from build123d import *

# Parameters (mm, degrees)
F2_SIZE  = 1.5
F3_W     = 30
F3_H     = 3
F4_DEPTH = 3.001


with BuildPart() as f1:
    # F0 (on Front) → F1 (revolve)
    with BuildSketch(Plane.XZ):
        Polygon((0, 10), (0, 15), (-3, 15), (-3, 0), (45, 0), (45, 10), (41.5, 10), (41.5, 7.5), (39.95, 7.5), (39.95, 10), align=None)
    revolve(axis=Axis((21, 0, 0), (1, 0, 0)))

    # F2
    f2_edges = [f1.edges().sort_by_distance(p)[0] for p in [
        (45, 0, -10),
        (-3, 0, -15),
    ]]
    chamfer(f2_edges, length=F2_SIZE)

    # F3 (on Right) → F4 (cut, through all)
    with BuildSketch(Plane.YZ):
        with Locations((0, 13.5)):
            Rectangle(F3_W, F3_H)
    extrude(amount=-F4_DEPTH, mode=Mode.SUBTRACT)


solid = f1.part
Input: part model. Units: mm. Frame: model coordinates. A direction names the side the tool comes from. Give positions to 0.01 mm unless a question says otherwise; leave off trailing zeros. Order: outer loops, then holes, each group sorted by start corner. A loop starts at its lowest first (then second) coordinate and runs counter-clockwise, first axis right, second up. Notation, with made-up numbers: (-31, 42.25) - (-6, 42.25) arc R38 ccw to (-6, 80.25) - close; hole circle Ø1 at (73.5, 43). An arc over 180 degrees is marked (long way). Answer as a JSON object with one key per item and string values. Group by question number.
Q1. Line query: probe 1 along X at (y, z) = (1, 8.25); probe 2 along X at (y, z) = (9, 1.25); probe 3 along Z at (x, y) = (10.5, 0.25). Output: solid intervals per line, ascending.
Q2. Cut plane A-A, the plane y = 0. Output: boundary loops of the cut face in (x, z).
Q3. Set-up query: faces 1 (the face through (19.7, 9.76, -2.17)), 2 (the face through (39.95, -7, -4)), 3 (the face through (-3, 0, -1)). Return all of +Z, -Z, +X, -X, +Y, -Y with unobstructed straight access to the full face (end or side cutting, diameter ignored); none if empty.
Q4. First-contact query: pin 1 Ø2 at (y, z) = (-7.5, 9) entering from +X; pin 2 Ø10 at (x, y) = (6, -1) entering from +Z; pin 3 Ø6 at (x, z) = (26, -3) entering from +Y. Flat tips, straight axial feed; report the tip coordinate or a pass-through.
Q5. Cut plane C-C, the plane x = 11.5. Output: boundary loops of the cut face in (y, z).
Q6. Mould query, pull axis X, two halves, no side actions, for faces 4 (the face through (40.714, -0.33, -7.493)), 5 (the face through (-2.76, -0.51, -13.73)), 6 (the face through (41.5, -7, 4)), 7 (the face through (42.49, 9.76, -2.17)). Classes: pulls with the +X half, pulls with the -X half, needs draft (parallel to the pull), parting line crosses it, or undercut.
Q7. Cut plane B-B, the plane z = 0. Output: boundary loops of the cut face in (x, y).
Results:
{
 "1": {"probe 1": "-3 to 39.95, 41.5 to 45", "probe 2": "-3 to 39.95, 41.5 to 44.41", "probe 3": "-10 to 10"},
 "2": {"outline": "(-3, -13.5) - (-1.5, -15) - (0, -15) - (0, -10) - (39.95, -10) - (39.95, -7.5) - (41.5, -7.5) - (41.5, -10) - (43.5, -10) - (45, -8.5) - (45, 8.5) - (43.5, 10) - (41.5, 10) - (41.5, 7.5) - (39.95, 7.5) - (39.95, 10) - (0, 10) - (0, 12) - (-3, 12) - close"},
 "3": {"face 1": "+X", "face 2": "none", "face 3": "+Z, -Z, -X, +Y, -Y"},
 "4": {"pin 1": "x = 0", "pin 2": "z = 10", "pin 3": "y = 10"},
 "5": {"outline": "circle Ø20 at (0, 0)"},
 "6": {"face 4": "undercut", "face 5": "pulls with the -X half", "face 6": "undercut", "face 7": "needs draft"},
 "7": {"outline": "(-3, -13.5) - (-1.5, -15) - (0, -15) - (0, -10) - (39.95, -10) - (39.95, -7.5) - (41.5, -7.5) - (41.5, -10) - (43.5, -10) - (45, -8.5) - (45, 8.5) - (43.5, 10) - (41.5, 10) - (41.5, 7.5) - (39.95, 7.5) - (39.95, 10) - (0, 10) - (0, 15) - (-1.5, 15) - (-3, 13.5) - close"}
}
